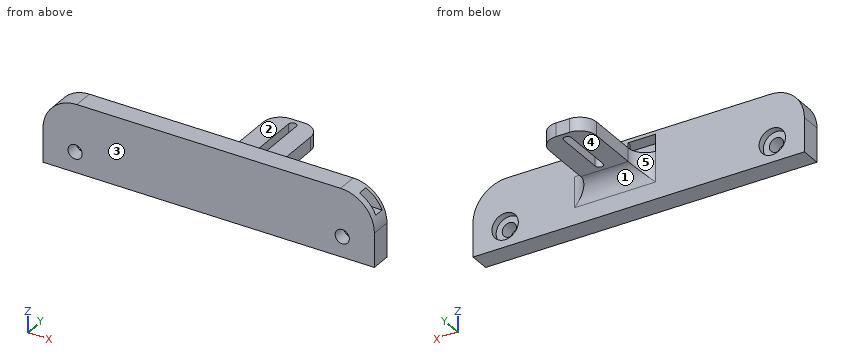
from build123d import *

# Parameters (mm, degrees)
CROQUIS1_R              = 2.1
SALIENTE_EXTRUIR1_DEPTH = 6
CROQUIS2_R              = 3.9
CORTAR_EXTRUIR1_DEPTH   = 2
CROQUIS3_W              = 14
CROQUIS3_H              = 4
SALIENTE_EXTRUIR2_DEPTH = 25
REDONDEO4_R             = 5
CORTAR_EXTRUIR6_DEPTH   = 4
REDONDEO7_R             = 5
REDONDEO8_R             = 5
CROQUIS5_W              = 5
CROQUIS5_H              = 8
CORTAR_EXTRUIR9_DEPTH   = 54
CROQUIS11_W             = 45
CROQUIS11_H             = 0.996592172
SALIENTE_EXTRUIR7_DEPTH = 5
CORTAR_EXTRUIR10_START  = -5
CORTAR_EXTRUIR10_DEPTH  = 5


with BuildPart() as part:
    # Croquis1 → Saliente-Extruir1 (new body)
    with BuildSketch(Plane(origin=(0, 0, 0), x_dir=(1, 0, 0), z_dir=(0, 1, 0))):
        with BuildLine():
            Line((-39, -10), (39, -10))
            ThreePointArc((39, -10), (46.071067812, -7.071067812), (49, 0))
            Line((49, 0), (49, 10))
            Line((49, 10), (-49, 10))
            Line((-49, 10), (-49, 0))
            ThreePointArc((-49, 0), (-46.071067812, -7.071067812), (-39, -10))
        make_face()
        with Locations(Location((-39.5, 4, 0), (0, 0, 270))):
            Circle(CROQUIS1_R, mode=Mode.SUBTRACT)
        with Locations(Location((39.5, 4, 0), (0, 0, 270))):
            Circle(CROQUIS1_R, mode=Mode.SUBTRACT)
    extrude(amount=SALIENTE_EXTRUIR1_DEPTH)

    # Croquis2 → Cortar-Extruir1 (cut)
    with BuildSketch(Plane(origin=(0, 6, 0), x_dir=(1, 0, 0), z_dir=(0, 1, 0))):
        with Locations(Location((39.5, 4, 0), (0, 0, 270))):
            Circle(CROQUIS2_R)
        with Locations(Location((-39.5, 4, 0), (0, 0, 270))):
            Circle(CROQUIS2_R)
    extrude(amount=-CORTAR_EXTRUIR1_DEPTH, mode=Mode.SUBTRACT)

    # Croquis3 → Saliente-Extruir2 (add)
    with BuildSketch(Plane(origin=(0, 6, 0), x_dir=(1, 0, 0), z_dir=(0, 1, 0))):
        with Locations((7, -2)):
            Rectangle(CROQUIS3_W, CROQUIS3_H)
    extrude(amount=SALIENTE_EXTRUIR2_DEPTH)

    # Redondeo4
    redondeo4_edges = [part.edges().sort_by_distance(p)[0] for p in [
        (7, 6, 0),
        (0, 6, 2),
        (14, 6, 2),
    ]]
    fillet(redondeo4_edges, radius=REDONDEO4_R)

    # Croquis4 → Cortar-Extruir6 (cut)
    with BuildSketch(Plane(origin=(0, 0, 0), x_dir=(-1, 0, 0), z_dir=(0, 0, -1))):
        with BuildLine():
            Line((-5.9, 28.5), (-5.9, 13.5))
            ThreePointArc((-5.9, 13.5), (-7.05, 12.35), (-8.2, 13.5))
            Line((-8.2, 13.5), (-8.2, 28.5))
            ThreePointArc((-8.2, 28.5), (-7.05, 29.65), (-5.9, 28.5))
        make_face()
    extrude(amount=-CORTAR_EXTRUIR6_DEPTH, mode=Mode.SUBTRACT)

    # Redondeo7
    redondeo7_edges = [part.edges().sort_by_distance(p)[0] for p in [
        (14, 31, 2),
    ]]
    fillet(redondeo7_edges, radius=REDONDEO7_R)

    # Redondeo8
    redondeo8_edges = [part.edges().sort_by_distance(p)[0] for p in [
        (0, 31, 2),
    ]]
    fillet(redondeo8_edges, radius=REDONDEO8_R)

    # Croquis5 → Cortar-Extruir9 (cut)
    with BuildSketch(Plane(origin=(49, 0, 0), x_dir=(0, 0, -1), z_dir=(1, 0, 0))):
        with Locations((-6.5, 6)):
            Rectangle(CROQUIS5_W, CROQUIS5_H)
    extrude(amount=-CORTAR_EXTRUIR9_DEPTH, mode=Mode.SUBTRACT)

    # Croquis11 → Saliente-Extruir7 (add)
    with BuildSketch(Plane.XY.offset(4)):
        with Locations((25.66515139, 5.501703914)):
            Rectangle(CROQUIS11_W, CROQUIS11_H)
    extrude(amount=SALIENTE_EXTRUIR7_DEPTH)

    # Croquis12 → Cortar-Extruir10 (cut)
    with BuildSketch(Plane(origin=(0, 6, 0), x_dir=(1, 0, 0), z_dir=(0, 1, 0)).offset(CORTAR_EXTRUIR10_START)):
        with BuildLine():
            Line((49, 10), (57.140229863, 10))
            Line((57.140229863, 10), (57.737940114, -14.066484251))
            Line((57.737940114, -14.066484251), (14, -12.561195781))
            Line((14, -12.561195781), (14, -10))
            Line((14, -10), (39, -10))
            ThreePointArc((39, -10), (46.071067812, -7.071067812), (49, 0))
            Line((49, 0), (49, 10))
        make_face()
    extrude(amount=CORTAR_EXTRUIR10_DEPTH, mode=Mode.SUBTRACT)


solid = part.part
Geometry: final body of the model. Coordinates: model frame, mm. Face numbers are marked on the shaded views. A direction names the side the tool comes from. Round coordinates to 2 decimals unless told otherwise and drop trailing zeros. Order: outer loops, then holes, each group sorted by start corner. A loop starts at its lowest first (then second) coordinate and runs counter-clockwise, first axis right, second up. Notation, with made-up numbers: (-32.75, 45.25) - (6.25, 45.25) arc R16 cw to (6.25, 68.25) - close; hole circle Ø6 at (27.25, -26.75). An arc over 180 degrees is marked (long way). Write each question's results on one line, items separated by ' | '.
Item 1: First-contact query: pin 1 Ø3.5 at (x, z) = (-39.5, -4) entering from +Y; pin 2 Ø3 at (y, z) = (20, 2.5) entering from -X; pin 3 Ø1.1 at (y, z) = (5.5, 7) entering from -X; pin 4 Ø3 at (y, z) = (4.5, 6) entering from +X. Flat tips, straight axial feed; report the tip coordinate or a pass-through.
Completed:
pin 1: through | pin 2: x = 0 | pin 3: x = -46.64 | pin 4: x = 47.89
Item 2: Section D-D, the plane z = 1.5. Return the cut outline in (x, y).
Completed:
outline: (-48.89, 0) - (48.89, 0) - (48.89, 6) - (19, 6) arc R5 cw to (14, 11) - (14, 26) arc R5 ccw to (9, 31) - (5, 31) arc R5 ccw to (0, 26) - (0, 11) arc R5 cw to (-5, 6) - (-48.89, 6) - close; hole (5.9, 13.5) arc R1.15 ccw to (8.2, 13.5) - (8.2, 28.5) arc R1.15 ccw to (5.9, 28.5) - close
Item 3: Material intervals for line 1 along X through (y, z) = (5.25, -4); line 2 along X through (y, z) = (2.4, -4); line 3 along Z through (x, y) = (-39.5, 3), sorted ascending. Write a range as [from, to].
Completed:
line 1: [-49, -43.4], [-35.6, 35.6], [43.4, 49] | line 2: [-49, -41.6], [-37.4, 37.4], [41.6, 49] | line 3: [-10, -6.1], [-1.9, 9.99]
Item 4: Section C-C, the plane x = 27. Return the cut outline in (y, z).
Completed:
outline: (0, -10) - (6, -10) - (6, 10) - (0, 10) - close; hole (2, 4) - (5, 4) - (5, 9) - (2, 9) - close
Item 5: Mould query, pull axis Z, two halves, no side actions, for the marked faces 1, 2 and 3. Classes: pulls with the +Z half, pulls with the -Z half, needs draft (parallel to the pull), parting line crosses it, or undercut.
Completed:
face 1: pulls with the -Z half | face 2: undercut | face 3: needs draft
Item 6: Reachability of the marked faces 4 and 5 from +Z, -Z, +X, -X, +Y, -Y: full face, straight path, thin tool, end or side. Return the list, or none.
Completed:
face 4: -Z, +X, -X, +Y | face 5: +Z, -Z, -X, +Y
Item 7: Section B-B, the plane y = 15. Return the cut outline in (x, z).
Completed:
outline: (0, 0) - (5.9, 0) - (5.9, 4) - (0, 4) - close; (8.2, 0) - (14, 0) - (14, 4) - (8.2, 4) - close
Item 8: Section A-A, the plane x = 7.05. Return the cut outline in (y, z).
Completed:
outline: (0, -10) - (6, -10) - (6, -5) arc R5 cw to (11, 0) - (12.35, 0) - (12.35, 4) - (6, 4) - (6, 10) - (0, 10) - close; (29.65, 0) - (31, 0) - (31, 4) - (29.65, 4) - close; hole (2, 4) - (5, 4) - (5, 9) - (2, 9) - close
